For this review, use the dimensioned drawing (mm, ordinates from the lowest corner) and the shaded views. A direction names the side the tool comes from. Coordinates: 2 decimals unless noted, no trailing zeros. Loops run counter-clockwise (first coordinate to the right, second up) from the corner with the lowest first, then second, coordinate; pieces in that order, holes last. Notation, with made-up numbers: (-3, 18) -> (1, 18) arc R9 cw to (1, 27) -> close; hole circle Ø1 at (58.5, 36). An arc over 180 degrees is marked (long way). Use one line per item in the form item = value. Start each with the question number.
1. Consider section A-A (x = 44). State the section outline as (y, z) points, then the cut area to 3 significant figures.
2. For pin 1 (5 mm diameter, centred on x = 71, z = 39.5, fed in from -Y); pin 2 (2 mm diameter, centred on y = 32.5, z = 64, fed in from -X); pin 3 (10 mm diameter, centred on x = 62, y = 77, fed in from +Z); pin 4 (1 mm diameter, centred on x = 71, y = 69.5, fed in from -Z), all flat-tipped, find the tip position at first contact; note any pin that passes through.
3. Consider section D-D (x = 7). State the section outline as (y, z) points, then the cut area to 3 significant figures.
4. Wall thickness on line 1 (Z direction, x = 82.5, y = 38); line 2 (Z direction, x = 44.5, y = 31); line 3 (X direction, y = 44.5, z = 42): over which ranges is each line inside the solid? List them lowest first. Write a range as from..to.
5. Machinability: for the marked faces 1, 2 and 3, which of the approach directions +Z, -Z, +X, -X, +Y, -Y give a long, thin tool a straight path to every point of the face, cutting with its end or side? Answer none if there is none.
6. Consider section C-C (y = 10). State the section outline as (x, z) points.
7. The part is to be moulded in two halves that separate along Z. For the marked faces 4, 5, 6 and 7, say which applies: released by +Z, released by -Z, zero draft, split by the parting line, or undercut.
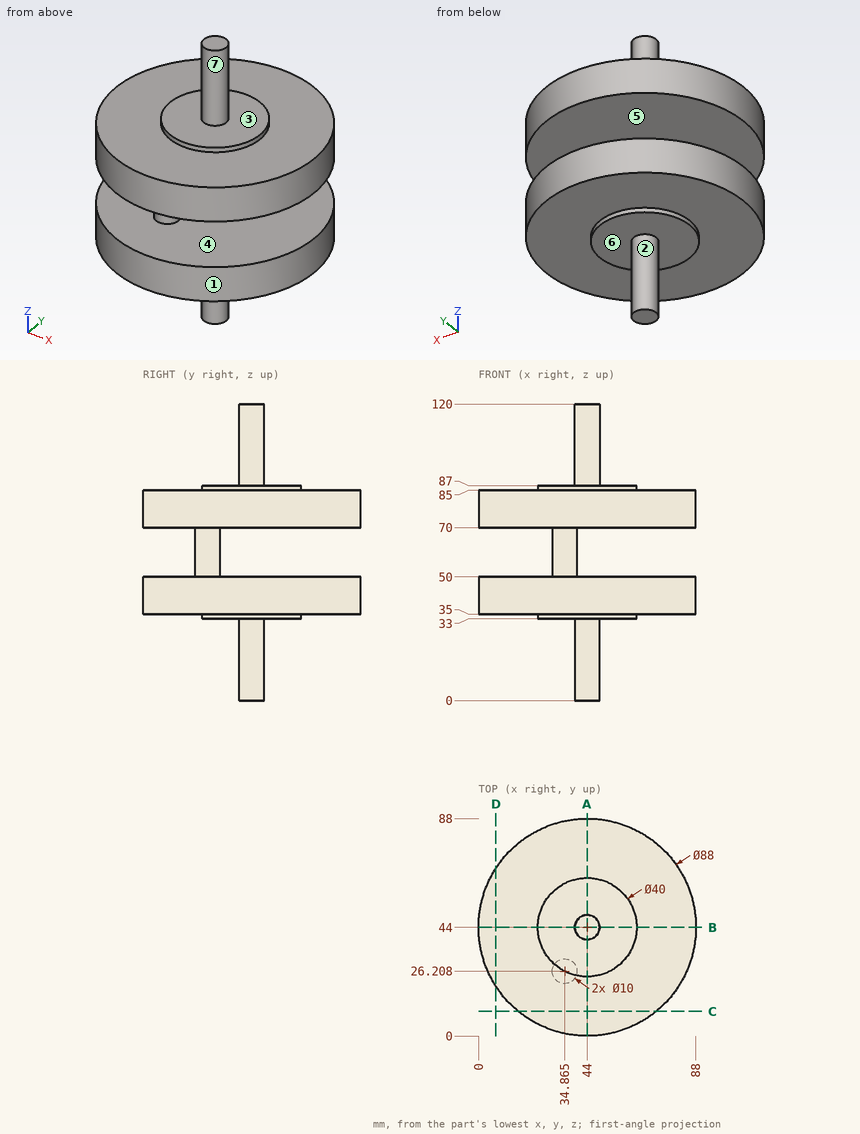
Geometry check:
q1.outline = (0, 35) -> (24, 35) -> (24, 33) -> (39, 33) -> (39, 0) -> (49, 0) -> (49, 33) -> (64, 33) -> (64, 35) -> (88, 35) -> (88, 50) -> (0, 50) -> close; (0, 70) -> (88, 70) -> (88, 85) -> (64, 85) -> (64, 87) -> (49, 87) -> (49, 120) -> (39, 120) -> (39, 87) -> (24, 87) -> (24, 85) -> (0, 85) -> close
q1.area = 3,460 mm²
q2.pin_1 = 7.45
q2.pin_2 = through
q2.pin_3 = 85
q2.pin_4 = 35
q3.outline = (20.19, 35) -> (67.81, 35) -> (67.81, 50) -> (20.19, 50) -> close; (20.19, 70) -> (67.81, 70) -> (67.81, 85) -> (20.19, 85) -> close
q3.area = 1,430 mm²
q4.line_1 = 35..50, 70..85
q4.line_2 = 33..50, 70..87
q4.line_3 = 0..88
q5.face_1 = +Z, -Z
q5.face_2 = -Z
q5.face_3 = +Z
q6.outline = (16.07, 35) -> (71.93, 35) -> (71.93, 50) -> (16.07, 50) -> close; (16.07, 70) -> (71.93, 70) -> (71.93, 85) -> (16.07, 85) -> close
q7.face_4 = undercut
q7.face_5 = undercut
q7.face_6 = released by -Z
q7.face_7 = zero draft
